Input: part model. Units: mm. Frame: model coordinates. Face numbers are marked on the shaded views. Give positions to 0.01 mm unless a question says otherwise; leave off trailing zeros. Order: outer loops, then holes, each group sorted by start corner. A loop starts at its lowest first (then second) coordinate and runs counter-clockwise, first axis right, second up. Notation, with made-up numbers: (-1, -26) -> (12, -26) arc R20 cw to (12, -19) -> close; hole circle Ø6 at (-1.5, -27). An arc over 180 degrees is marked (long way). Use a Markdown table: item, result. Add a question column.
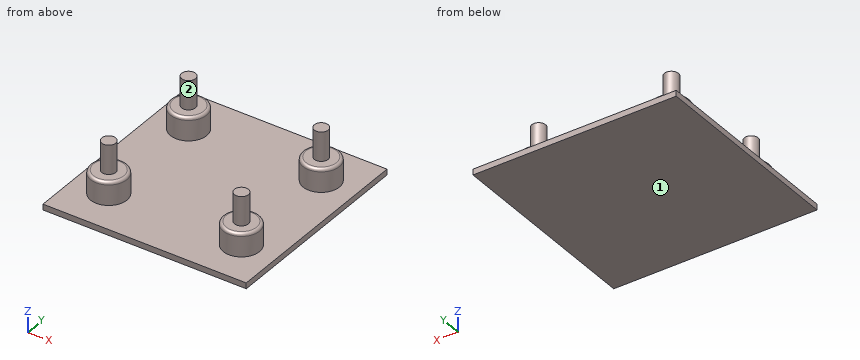
Autodesk Inventor part; units mm, degrees
ref_plane "Work Plane1" through (0, 0, 3.85) normal (0, 0, 1) x (1, 0, 0)
ref_plane "YZ Plane" through (0, 0, 0) normal (1, 0, 0) x (0, 1, 0)
ref_plane "XZ Plane" through (0, 0, 0) normal (0, 1, 0) x (-1, 0, 0)
ref_plane "Work Plane1" through (0, 0, 3.85) normal (0, 0, 1) x (1, 0, 0)
sketch "Sketch1" plane through (0, 0, 3.85) normal (0, 0, 1) x (1, 0, 0)
  line L0 (-150, -25) -> (-80, -25)
  line L1 (-80, -25) -> (-80, 45)
  line L2 (-80, 45) -> (-150, 45)
  line L3 (-150, 45) -> (-150, -25)
  circle A0 centre (-10, 10) radius 2.5
  line L4 (-150, 0) -> (-150, 5.1)
  line L5 (-150, 14.9) -> (-150, 20)
  point P0 (0, 0)
  dimension "d0" = 70
  dimension "d20" = 70
  dimension "d21" = 0
extrude "Extrusion1" add sketch "Sketch1" along normal blind 2 contours L3 L2 L1 L0
sketch "Sketch2" plane through (0, 0, 5.85) normal (0, 0, 1) x (1, 0, 0)
  line L0 (-80, -25) -> (-80, 45)
  line L1 (-80, 45) -> (-150, 45)
  line L2 (-150, 45) -> (-150, -25)
  line L3 (-150, -25) -> (-80, -25)
  circle A0 centre (-137.85, -9.85) radius 2.4
  circle A1 centre (-137.85, 29.85) radius 2.4
  circle A2 centre (-92.15, -9.85) radius 2.4
  circle A3 centre (-92.15, 29.85) radius 2.4
  line L4 (-140.25, -12.25) -> (-89.75, -12.25)
  line L5 (-89.75, -12.25) -> (-89.75, 32.25)
  line L6 (-89.75, 32.25) -> (-140.25, 32.25)
  line L7 (-140.25, 32.25) -> (-140.25, -12.25)
  line L8 (-150, -25) -> (-80, 45) construction
  line L9 (-80, -25) -> (-150, 45) construction
  line L10 (-89.75, -12.25) -> (-140.25, 32.25) construction
  line L11 (-140.25, -12.25) -> (-89.75, 32.25) construction
  point P0 (0, 0)
  point P1 (-115, 10)
  dimension "d5" = 4.8
  dimension "d6" = 4.8
  dimension "d7" = 4.8
  dimension "d8" = 4.8
  dimension "d9" = 44.5
  dimension "d10" = 50.5
extrude "Extrusion2" add sketch "Sketch2" along normal blind 18 contours A0 | A1 | A2 | A3
sketch "Sketch3" plane through (0, 0, 5.85) normal (0, 0, 1) x (1, 0, 0)
  circle A0 centre (-92.15, -9.85) radius 2.4
  circle A1 centre (-92.15, 29.85) radius 2.4
  circle A2 centre (-137.85, -9.85) radius 2.4
  circle A3 centre (-137.85, 29.85) radius 2.4
  circle A4 centre (-137.85, -9.85) radius 6.25
  circle A5 centre (-137.85, 29.85) radius 6.25
  circle A6 centre (-92.15, -9.85) radius 6.25
  circle A7 centre (-92.15, 29.85) radius 6.25
  point P0 (0, 0)
  dimension "d13" = 12.5
  dimension "d14" = 12.5
  dimension "d15" = 12.5
  dimension "d16" = 12.5
extrude "Extrusion3" add sketch "Sketch3" along normal blind 8
fillet "Fillet1" radius 1 4 edges at (-144.1, -9.85, 13.85) (-98.4, -9.85, 13.85) (-98.4, 29.85, 13.85) (-144.1, 29.85, 13.85)
equation "\"d20\" = d0"
equation "\"d14\" = d13"
equation "\"d15\" = d13"
equation "\"d16\" = d13"
properties part number "Plateo"
Q1. Section query B-B (y = -9.85). Return loops of the section in (x, z), plus the area to 3 significant figures.
Q2. Ray query, line 1 (Z direction, x = -94, y = -19.5); line 2 (Z direction, x = -88.5, y = 33.5); line 3 (X direction, y = 26, z = 8.5). Return the intervals inside material, ascending.
Q3. First-contact query: pin 1 (2 mm diameter, centred on x = -95, z = 13, fed in from -Y); pin 2 (5 mm diameter, centred on y = -13, z = 15.5, fed in from -X); pin 3 (6 mm diameter, centred on x = -141, z = 9.5, fed in from -Y). Flat tips, straight axial feed; report the tip coordinate or a pass-through.
Q4. Section query D-D (z = 9). Return loops of the section in (x, y).
Q5. Section query C-C (z = 15.25). Return loops of the section in (x, y).
Q6. Draft query along X for the marked faces 1 and 2. Return one class per face: +X half, -X half, draft (parallel to the pull), parting line (faces both ways), or undercut.
Q7. Section query A-A (x = -137.85). Return loops of the section in (y, z), plus the area to 3 significant figures.
Solution:
| question | item | result |
|---|---|---|
| 1 | outline | (-150, 3.85) -> (-80, 3.85) -> (-80, 5.85) -> (-85.9, 5.85) -> (-85.9, 12.85) arc R1 ccw to (-86.9, 13.85) -> (-89.75, 13.85) -> (-89.75, 23.85) -> (-94.55, 23.85) -> (-94.55, 13.85) -> (-97.4, 13.85) arc R1 ccw to (-98.4, 12.85) -> (-98.4, 5.85) -> (-131.6, 5.85) -> (-131.6, 12.85) arc R1 ccw to (-132.6, 13.85) -> (-135.45, 13.85) -> (-135.45, 23.85) -> (-140.25, 23.85) -> (-140.25, 13.85) -> (-143.1, 13.85) arc R1 ccw to (-144.1, 12.85) -> (-144.1, 5.85) -> (-150, 5.85) -> close |
| 1 | area | 435 mm² |
| 2 | line 1 | z = 3.85 to 5.85 |
| 2 | line 2 | z = 3.85 to 13.85 |
| 2 | line 3 | x = -142.77 to -132.93, -97.07 to -87.23 |
| 3 | pin 1 | stops at y = -15.82 |
| 3 | pin 2 | stops at x = -143.67 |
| 3 | pin 3 | stops at y = -16.1 |
| 4 | outline | circle Ø12.5 at (-137.85, -9.85); circle Ø12.5 at (-137.85, 29.85); circle Ø12.5 at (-92.15, -9.85); circle Ø12.5 at (-92.15, 29.85) |
| 5 | outline | circle Ø4.8 at (-137.85, -9.85); circle Ø4.8 at (-137.85, 29.85); circle Ø4.8 at (-92.15, -9.85); circle Ø4.8 at (-92.15, 29.85) |
| 6 | face 1 | draft |
| 6 | face 2 | undercut |
| 7 | outline | (-25, 3.85) -> (45, 3.85) -> (45, 5.85) -> (36.1, 5.85) -> (36.1, 12.85) arc R1 ccw to (35.1, 13.85) -> (32.25, 13.85) -> (32.25, 23.85) -> (27.45, 23.85) -> (27.45, 13.85) -> (24.6, 13.85) arc R1 ccw to (23.6, 12.85) -> (23.6, 5.85) -> (-3.6, 5.85) -> (-3.6, 12.85) arc R1 ccw to (-4.6, 13.85) -> (-7.45, 13.85) -> (-7.45, 23.85) -> (-12.25, 23.85) -> (-12.25, 13.85) -> (-15.1, 13.85) arc R1 ccw to (-16.1, 12.85) -> (-16.1, 5.85) -> (-25, 5.85) -> close |
| 7 | area | 435 mm² |
